Could you check a few things on this model? Use its own coordinates, in mm. A direction names the side the tool comes from. Coordinates: 2 decimals unless noted, no trailing zeros. Order: outer loops, then holes, each group sorted by start corner. A loop starts at its lowest first (then second) coordinate and runs counter-clockwise, first axis right, second up. Notation, with made-up numbers: M 51.5,-29 L 72.5,-29 A18 ccw 72.5,-12 Z; hole C 43,66 d4. An arc over 180 degrees is marked long. Write item = value, one per line. Start each with the question number.
Autodesk Inventor part; units mm, degrees
ref_plane "YZ Plane" through (0, 0, 0) normal (1, 0, 0) x (0, 1, 0)
ref_plane "XZ Plane" through (0, 0, 0) normal (0, 1, 0) x (-1, 0, 0)
ref_plane "XY Plane" through (0, 0, 0) normal (0, 0, 1) x (1, 0, 0)
sketch "Sketch1" plane through (0, 0, 0) normal (0, 1, 0) x (-1, 0, 0)
  line L0 (-75, 75) -> (75, 75)
  line L1 (75, 75) -> (75, -75)
  line L2 (75, -75) -> (-75, -75)
  line L3 (-75, -75) -> (-75, 75)
  line L4 (-75, 75) -> (75, -75) construction
  line L5 (75, 75) -> (-75, -75) construction
  circle A0 centre (0, 0) radius 60
  line L6 (-62.5, 62.5) -> (62.5, 62.5) construction
  line L7 (62.5, 62.5) -> (62.5, -62.5) construction
  line L8 (62.5, -62.5) -> (-62.5, -62.5) construction
  line L9 (-62.5, -62.5) -> (-62.5, 62.5) construction
  line L10 (-62.5, 62.5) -> (62.5, -62.5) construction
  line L11 (62.5, 62.5) -> (-62.5, -62.5) construction
  circle A1 centre (62.5, 62.5) radius 2.5
  circle A2 centre (62.5, -62.5) radius 2.5
  circle A3 centre (-62.5, 62.5) radius 2.5
  circle A4 centre (-62.5, -62.5) radius 2.5
  line L12 (64.6213, -64.6213) -> (60.3787, -60.3787) construction
  line L13 (62.8536, -66.3891) -> (58.6109, -62.1464)
  line L14 (62.1464, -58.6109) -> (66.3891, -62.8536)
  arc A5 (62.8536, -66.3891) -> (66.3891, -62.8536) centre (64.6213, -64.6213) ccw
  arc A6 (62.1464, -58.6109) -> (58.6109, -62.1464) centre (60.3787, -60.3787) ccw
  line L15 (-64.6213, -64.6213) -> (-60.3787, -60.3787) construction
  line L16 (-62.8536, -66.3891) -> (-58.6109, -62.1464)
  line L17 (-62.1464, -58.6109) -> (-66.3891, -62.8536)
  arc A7 (-66.3891, -62.8536) -> (-62.8536, -66.3891) centre (-64.6213, -64.6213) ccw
  arc A8 (-58.6109, -62.1464) -> (-62.1464, -58.6109) centre (-60.3787, -60.3787) ccw
  line L18 (-64.6213, 64.6213) -> (-60.3787, 60.3787) construction
  line L19 (-62.8536, 66.3891) -> (-58.6109, 62.1464)
  line L20 (-62.1464, 58.6109) -> (-66.3891, 62.8536)
  arc A9 (-62.8536, 66.3891) -> (-66.3891, 62.8536) centre (-64.6213, 64.6213) ccw
  arc A10 (-62.1464, 58.6109) -> (-58.6109, 62.1464) centre (-60.3787, 60.3787) ccw
  line L21 (64.6213, 64.6213) -> (60.3787, 60.3787) construction
  line L22 (62.8536, 66.3891) -> (58.6109, 62.1464)
  line L23 (62.1464, 58.6109) -> (66.3891, 62.8536)
  arc A11 (66.3891, 62.8536) -> (62.8536, 66.3891) centre (64.6213, 64.6213) ccw
  arc A12 (58.6109, 62.1464) -> (62.1464, 58.6109) centre (60.3787, 60.3787) ccw
  dimension "d0" = 150
  dimension "d1" = 150
  dimension "d2" = 120
  dimension "d3" = 125
  dimension "d4" = 5
  dimension "d5" = 5
  dimension "d6" = 5
  dimension "d7" = 5
  dimension "d21" = 3
  dimension "d22" = 3
  dimension "d23" = 3
  dimension "d24" = 3
extrude "Extrusion1" add sketch "Sketch1" along normal blind 3
sketch "Sketch2" plane through (0, 0, 0) normal (0, -1, 0) x (1, 0, 0)
  line L0 (-71.5, -71.5) -> (71.5, -71.5)
  line L1 (71.5, -71.5) -> (71.5, 71.5)
  line L2 (71.5, 71.5) -> (-71.5, 71.5)
  line L3 (-71.5, 71.5) -> (-71.5, -71.5)
  line L4 (-71.5, -71.5) -> (71.5, 71.5) construction
  line L5 (71.5, -71.5) -> (-71.5, 71.5) construction
  point P0 (0, 0)
  dimension "d11" = 143
  dimension "d19" = 143
hole "Hole1" at (-71.5, 0, 71.5) at (71.5, 0, 71.5) at (71.5, 0, -71.5) at (-71.5, 0, -71.5) direction (0, 1, 0) diameter 5.5 depth 6 tip angle 118
fillet "Fillet2" radius 2 4 edges at (-75, 1.5, 75) (75, 1.5, 75) (-75, 1.5, -75) (75, 1.5, -75)
equation "\"d8\" = d24"
properties part number "150mm_Bearing_Plate" material "Aluminum 6061"
(1) Imagine slicing it at B-B on z = 0. List the corners of the cut face in (x, y) for me.
(2) For faces 3 (the flat face through (34, 0, 51)), 4 (the flat face through (60.762, 1.479, -64.297)), which set-ups out of +Z, -Z, +X, -X, +Y, -Y let a thin tool reach every point of the face, with its end or its side?
(3) Imagine slicing it at A-A on y = 0.45. Give the number of separate pieces and of enclosed holes in the cut face, plus the area to 3 significant figures.
(4) Please list where these lines run through material, in increasing order: probe 1 along Z at (x, y) = (71.5, 1.85); probe 2 along Z at (x, y) = (66.5, 0.7). Write a range as from..to.
(5) Imagine slicing it at C-C on x = -36. List the corners of the cut face in (y, z) for me.
(6) Thinking about a two-plate mould opening in X: for faces 1 (the flat face through (34, 3, 51)), 2 (the cylindrical face through (69.641, 1.521, 73.527)), which applies, released by +X, released by -X, zero draft, split by the parting line, or undercut?
Response:
q1.outline = M -75,0 L -60,0 L -60,3 L -75,3 Z; M 60,0 L 75,0 L 75,3 L 60,3 Z
q2.face_3 = +Z, -Z, +X, -X, -Y
q2.face_4 = +Y, -Y
q3.separate_pieces = 1
q3.enclosed_holes = 9
q3.area = 10,900 mm2
q4.probe_1 = -75..-74.25, -68.75..68.75, 74.25..75
q4.probe_2 = -75..-66.27, -62.97..62.97, 66.27..75
q5.outline = M 0,-75 L 3,-75 L 3,-48 L 0,-48 Z; M 0,48 L 3,48 L 3,75 L 0,75 Z
q6.face_1 = zero draft
q6.face_2 = undercut
